For this review, take the finished solid that the model builds, in its own axes (mm). A direction names the side the tool comes from. Coordinates: 2 decimals unless noted, no trailing zeros. Loops run counter-clockwise (first coordinate to the right, second up) from the corner with the lowest first, then second, coordinate; pieces in that order, holes last. Notation, with made-up numbers: (80.5, 78.5) -> (121.5, 78.5) arc R26 cw to (121.5, 96.5) -> close; hole circle Ø4 at (-4.5, 32). An arc over 180 degrees is marked (long way). Use a Markdown table: item, result.
from build123d import *

# Parameters (mm, degrees)
F2_R             = 3.175
F3_R             = 3.175
F4_SIZE          = 3.175
F5_R             = 3.3147
F6_DEPTH         = 152.401
F6_COPIES_COUNT  = 6
F7_W             = 3.175
F7_H             = 3.175
F8_DEPTH         = 25.4
F9_R             = 4.8895
F10_DEPTH        = 152.401
F10_COPIES_COUNT = 4
F11_R            = 6.35
F12_DEPTH        = 6.35
F12_COPIES_COUNT = 4


# Not quite as in the source:
# - a pattern or mirror of a feature is missing from the dataset's text; its kind, count and spacing are read off the source's solid


with BuildPart() as f1:
    # F0 (on Front) → F1 (revolve)
    with BuildSketch(Plane.XZ):
        Polygon((0, 12.7), (0, 0), (152.4, 0), (152.4, 44.45), (139.7, 44.45), (139.7, 19.05), (50.8, 19.05), (50.8, 12.7), align=None)
    revolve(axis=Axis((76.2, 0, 0), (1, 0, 0)))

    # F2
    f2_edges = [f1.edges().sort_by_distance(p)[0] for p in [
        (50.8, 0, -12.7),
    ]]
    fillet(f2_edges, radius=F2_R)

    # F3
    f3_edges = [f1.edges().sort_by_distance(p)[0] for p in [
        (139.7, 0, -19.05),
    ]]
    fillet(f3_edges, radius=F3_R)

    # F4
    f4_edges = [f1.edges().sort_by_distance(p)[0] for p in [
        (0, 0, -12.7),
    ]]
    chamfer(f4_edges, length=F4_SIZE)

    # F5 (on face) → F6 (cut, through all)
    with BuildSketch(Plane.YZ.offset(152.4)):
        with Locations((0, -34.925)):
            Circle(F5_R)
    f6 = extrude(amount=-F6_DEPTH, mode=Mode.SUBTRACT)

    # F6_copies: F6 ×6 about axis
    f6_copies_axis = Axis((0, 0, 0), (1, 0, 0))
    for i in range(1, F6_COPIES_COUNT):
        add(f6.rotate(f6_copies_axis, i * 360 / F6_COPIES_COUNT), mode=Mode.SUBTRACT)

    # F7 (on face) → F8 (cut)
    with BuildSketch(Plane(origin=(50.8, 0, 0), x_dir=(0, -1, 0), z_dir=(-1, 0, 0))):
        with Locations((1.5875, -17.4625)):
            Rectangle(F7_W, F7_H)
        with Locations((-1.5875, -17.4625)):
            Rectangle(F7_W, F7_H)
    extrude(amount=-F8_DEPTH, mode=Mode.SUBTRACT)

    # F9 (on face) → F10 (cut, through all)
    with BuildSketch(Plane.YZ.offset(152.4)):
        with Locations((-20.2055762724, -20.2055762724)):
            Circle(F9_R)
    f10 = extrude(amount=-F10_DEPTH, mode=Mode.SUBTRACT)

    # F10_copies: F10 ×4 about axis
    f10_copies_axis = Axis((0, 0, 0), (1, 0, 0))
    for i in range(1, F10_COPIES_COUNT):
        add(f10.rotate(f10_copies_axis, i * 360 / F10_COPIES_COUNT), mode=Mode.SUBTRACT)

    # F11 (on face) → F12 (cut)
    with BuildSketch(Plane(origin=(139.7, 0, 0), x_dir=(0, -1, 0), z_dir=(-1, 0, 0))):
        with Locations((20.2055762724, -20.2055762724)):
            Circle(F11_R)
    f12 = extrude(amount=-F12_DEPTH, mode=Mode.SUBTRACT)

    # F12_copies: F12 ×4 about axis
    f12_copies_axis = Axis((0, 0, 0), (1, 0, 0))
    for i in range(1, F12_COPIES_COUNT):
        add(f12.rotate(f12_copies_axis, i * 360 / F12_COPIES_COUNT), mode=Mode.SUBTRACT)


solid = f1.part
(1) Take a section at C-C on y = -39. Write out the cut boundary in (x, z), plus the area to 3 significant figures.
Found:
| item | result |
|---|---|
| outline | (139.7, -21.33) -> (152.4, -21.33) -> (152.4, 21.33) -> (139.7, 21.33) -> close |
| area | 542 mm^2 |
(2) Mouldability with a two-part tool opening along Z and no side actions: class faces 3 (the face through (63, 0, -15.875)), 4 (the face through (142.83, -15.53, -15.91)), 5 (the face through (76.2, 0, -17)) as pulls with the +Z half, pulls with the -Z half, needs draft (parallel to the pull), parting line crosses it, or undercut.
Found:
| item | result |
|---|---|
| face 3 | pulls with the -Z half |
| face 4 | undercut |
| face 5 | needs draft |
(3) Take a section at B-B on x = 115. Write out the cut boundary in (y, z), plus the area to 3 significant figures.
Found:
| item | result |
|---|---|
| outline | circle Ø38.1 at (0, 0) |
| area | 1,140 mm^2 |
(4) Take a section at D-D on x = 66. Write out the cut boundary in (y, z) (3 decimals).
Found:
| item | result |
|---|---|
| outline | (-3.175, -18.784) -> (-3.175, -15.875) -> (3.175, -15.875) -> (3.175, -18.784) arc R19.05 ccw (long way) to start |
(5) For faces 1 (the face through (146.14, 0.72, 38.16)), 2 (the face through (146.05, 22, 25)), list the 3-axis set-ups (+Z, -Z, +X, -X, +Y, -Y) from which the entire face can be reached by the end or side of a thin tool; tool diameter is ignored.
Found:
| item | result |
|---|---|
| face 1 | +X, -X |
| face 2 | -X |
(6) For line 1 along Z through (x, y) = (143, 0); line 2 along Y through (x, z) = (141, 19); line 3 along X through (y, z) = (-33.5, 10), list the stretches that pass through material, from the lowest coordinate up.
Found:
| item | result |
|---|---|
| line 1 | z = -44.45 to -38.24, -31.61 to 31.61, 38.24 to 44.45 |
| line 2 | y = -40.18 to -33.18, -27.31 to -26.44, -13.97 to 13.97, 26.44 to 27.31, 33.18 to 40.18 |
| line 3 | x = 139.7 to 152.4 |
(7) Take a section at A-A on z = 0. Write out the cut boundary in (x, y) (3 decimals), plus the area to 4 significant figures.
Found:
| item | result |
|---|---|
| outline | (0, -9.525) -> (3.175, -12.7) -> (47.625, -12.7) arc R3.175 cw to (50.8, -15.875) -> (50.8, -19.05) -> (136.525, -19.05) arc R3.175 cw to (139.7, -22.225) -> (139.7, -44.45) -> (152.4, -44.45) -> (152.4, 44.45) -> (139.7, 44.45) -> (139.7, 22.225) arc R3.175 cw to (136.525, 19.05) -> (50.8, 19.05) -> (50.8, 15.875) arc R3.175 cw to (47.625, 12.7) -> (3.175, 12.7) -> (0, 9.525) -> close |
| area | 5,805 mm^2 |
(8) For pin 1 Ø2.5 at (x, z) = (65, -17.5) entering from +Y; pin 2 Ø12.5 at (y, z) = (20.21, 20.21) entering from +X; pin 3 Ø7.5 at (y, z) = (-30.25, 17.46) entering from -X; pin 4 Ø12 at (x, z) = (134, 21) entering from +Y, all flat-tipped, find the tip position at first contact; note any pin that passes through.
Found:
| item | result |
|---|---|
| pin 1 | stops at y = 9.94 |
| pin 2 | stops at x = 152.4 |
| pin 3 | stops at x = 139.7 |
| pin 4 | stops at y = 40.12 |
